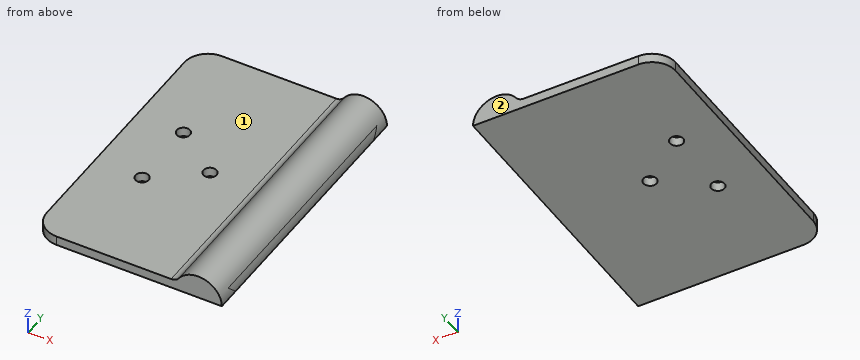
from build123d import *

# Parameters (mm, degrees)
SKETCH1_R           = 1.4
BOSS_EXTRUDE1_DEPTH = 2
BOSS_EXTRUDE2_DEPTH = 60
CUT_EXTRUDE1_DEPTH  = 60
FILLET1_R           = 2


with BuildPart() as part:
    # Sketch1 → Boss-Extrude1 (new body)
    with BuildSketch(Plane(origin=(0, 0, -2), x_dir=(-1, 0, 0), z_dir=(0, 0, -1))):
        with BuildLine():
            Line((60.9850693, 26.806434403), (30.9850693, 26.806434403))
            ThreePointArc((30.9850693, 26.806434403), (27.449535394, 25.341968309), (25.9850693, 21.806434403))
            Line((25.9850693, 21.806434403), (25.9850693, -28.193565597))
            ThreePointArc((25.9850693, -28.193565597), (27.449535394, -31.729099503), (30.9850693, -33.193565597))
            Line((30.9850693, -33.193565597), (60.9850693, -33.193565597))
            ThreePointArc((60.9850693, -33.193565597), (64.520603206, -31.729099503), (65.9850693, -28.193565597))
            Line((65.9850693, -28.193565597), (65.9850693, 21.806434403))
            ThreePointArc((65.9850693, 21.806434403), (64.520603206, 25.341968309), (60.9850693, 26.806434403))
        make_face()
        with Locations(Location((55.9850693, 4.306434403, 0), (0, 0, 180))):
            Circle(SKETCH1_R, mode=Mode.SUBTRACT)
        with Locations(Location((55.9850693, -10.693565597, 0), (0, 0, 180))):
            Circle(SKETCH1_R, mode=Mode.SUBTRACT)
        with Locations(Location((45.9850693, -3.193565597, 0), (0, 0, 180))):
            Circle(SKETCH1_R, mode=Mode.SUBTRACT)
    extrude(amount=-BOSS_EXTRUDE1_DEPTH)

    # Sketch2 → Boss-Extrude2 (add)
    with BuildSketch(Plane(origin=(0, 26.806434403, 0), x_dir=(1, 0, 0), z_dir=(0, 1, 0))):
        with BuildLine():
            Line((-25.9850693, 2), (-35.9850693, 2))
            ThreePointArc((-35.9850693, 2), (-30.9850693, -3), (-25.9850693, 2))
        make_face()
    extrude(amount=-BOSS_EXTRUDE2_DEPTH)

    # Sketch3 → Cut-Extrude1 (cut)
    with BuildSketch(Plane(origin=(0, 26.806434403, 0), x_dir=(1, 0, 0), z_dir=(0, 1, 0))):
        with BuildLine():
            Line((-26.402493605, 0), (-25.9850693, 0))
            Line((-25.9850693, 0), (-25.9850693, 2))
            ThreePointArc((-25.9850693, 2), (-26.090537735, 0.978451782), (-26.402493605, 0))
        make_face()
    extrude(amount=-CUT_EXTRUDE1_DEPTH, mode=Mode.SUBTRACT)

    # Fillet1
    fillet1_edges = [part.edges().sort_by_distance(p)[0] for p in [
        (-35.567644995, -3.193565597, 0),
    ]]
    fillet(fillet1_edges, radius=FILLET1_R)


solid = part.part
Work out the finished part from the listing and answer in its coordinate system (mm). Face numbers are marked on the shaded views. A direction names the side the tool comes from. Give positions to 0.01 mm unless a question says otherwise; leave off trailing zeros. Order: outer loops, then holes, each group sorted by start corner. A loop starts at its lowest first (then second) coordinate and runs counter-clockwise, first axis right, second up. Notation, with made-up numbers: (42.5, 26.25) -> (96.5, 26.25) arc R18 ccw to (96.5, 58.25) -> close; hole circle Ø4 at (-9, 85). An arc over 180 degrees is marked (long way). Answer as a JSON object with one key per item and string values. Group by question number.
1. A tool of negligible diameter and unlimited length cuts with its end or side. For the marked faces 1 and 2, from which of +Z, -Z, +X, -X, +Y, -Y can it reach the whole face along a straight path? Write none if from no direction.
2. Section D-D on z = 2.1 is taken. Determine the outline of the cut face in (x, y).
3. Section C-C on y = -26 is taken. Determine the outline of the cut face in (x, z).
4. Consider line 1 along Y through (x, z) = (-46, -1.25); line 2 along Z through (x, y) = (-54, -26); line 3 along Z through (x, y) = (-30.5, 15.5). Determine where each line is inside the solid, lowest interval first. Write a range as [from, to].
5. Section A-A on x = -56 is taken. Determine the outline of the cut face in (y, z).
6. Section B-B on y = -10 is taken. Determine the outline of the cut face in (x, z), plus the area to 3 significant figures.
7. Flat-ended cylindrical pins translate along their axes: pin 1 Ø5 at (x, y) = (-39, -21.5) entering from +Z; pin 2 Ø4.5 at (x, y) = (-55.99, 4.31) entering from -Z; pin 3 Ø1.5 at (x, z) = (-62, 0.5) entering from +Y. Find the tip coordinate at first contact, or state that the pin passes through.
Result sheet:
{
 "1": {"face 1": "+Z, -X, +Y, -Y", "face 2": "+Z, -Z, +X, -X, +Y"},
 "2": {"outline": "(-33.85, -33.19) -> (-28.12, -33.19) -> (-28.12, 26.81) -> (-33.85, 26.81) -> close"},
 "3": {"outline": "(-65.99, -2) -> (-25.99, -2) arc R5 ccw to (-35.09, 0.86) arc R2 cw to (-36.73, 0) -> (-65.99, 0) -> close"},
 "4": {"line 1": "y = [-33.19, -4.59], [-1.79, 26.81]", "line 2": "z = [-2, 0]", "line 3": "z = [-2, 2.98]"},
 "5": {"outline": "(-33.19, -2) -> (-12.09, -2) -> (-12.09, 0) -> (-33.19, 0) -> close; (-9.29, -2) -> (2.91, -2) -> (2.91, 0) -> (-9.29, 0) -> close; (5.71, -2) -> (26.81, -2) -> (26.81, 0) -> (5.71, 0) -> close"},
 "6": {"outline": "(-65.99, -2) -> (-57.2, -2) -> (-57.2, 0) -> (-65.99, 0) -> close; (-54.77, -2) -> (-25.99, -2) arc R5 ccw to (-35.09, 0.86) arc R2 cw to (-36.73, 0) -> (-54.77, 0) -> close", "area": "94.9 mm^2"},
 "7": {"pin 1": "stops at z = 0.01", "pin 2": "stops at z = -2", "pin 3": "stops at y = 26.79"}
}
